Part model, mm, in its own coordinate system. A direction names the side the tool comes from. Round coordinates to 2 decimals unless told otherwise and drop trailing zeros. Loops run counter-clockwise (first coordinate to the right, second up) from the corner with the lowest first, then second, coordinate; pieces in that order, holes last.
(1) Probe probe 1 along X at (y, z) = (-0.3, 0); probe 2 along X at (y, z) = (-2.5, 0); probe 3 along Y at (x, z) = (-8.5, 2). List the from-to ranges inside material, lowest first.
(2) Mould opens along Z. For faces 3 (the face through (0, -1, -5.85)), 4 (the face through (-0.976, -0.507, 0.217)), 5 (the face through (2, -1.95, -4)) say: +Z half, -Z half, draft (parallel to the pull), parting line (faces both ways), or undercut.
(3) Flat gauge pins, fed straight in: pin 1 (3 mm diameter, centred on y = -1, z = 2.5, fed in from +X); pin 2 (1 mm diameter, centred on y = -3.5, z = 2, fed in from +X); pin 3 (3 mm diameter, centred on x = -0.5, z = -1, fed in from -Y). Where does each tip first touch, or does it go through?
(4) Cut at B-B on z = 0. List the corners of the cut face in (x, y).
(5) Tool access for faces 1 (the face through (0, -1, -1.2)), 2 (the face through (11, -1, 0)): list every direction of +Z, -Z, +X, -X, +Y, -Y with a clear straight run to the whole face (end or side of a thin tool).
(6) Cut at C-C on y = -4.95. List the corners of the cut face in (x, z), then the cut area to 3 significant figures.
(7) Cut at D-D on z = -1.5. List the corners of the cut face in (x, y), then the cut area to 3 significant figures.
(8) Cut at A-A on x = 0. List the corners of the cut face in (y, z), then the cut area to 3 significant figures.
from build123d import *

# Parameters (mm, degrees)
BOSS_EXTRUDE1_DEPTH     = 1.95
SKETCH2_R               = 4
BOSS_EXTRUDE2_DEPTH     = 3.55
SKETCH3_R               = 2.86
CUT_EXTRUDE1_DEPTH      = 4.5
SKETCH4_R               = 1
CUT_EXTRUDE2_DEPTH      = 1
CUT_EXTRUDE3_DEPTH      = 25.219723368
CUT_EXTRUDE3_DEPTH_BACK = 25.219723368
SKETCH5_OUTSIDE_W       = 57.198
SKETCH5_OUTSIDE_H       = 23.198
SKETCH5_OUTSIDE_R       = 11


with BuildPart() as part:
    # Sketch1 → Boss-Extrude1 (new body)
    with BuildSketch(Plane(origin=(0, 0, 0), x_dir=(1, 0, 0), z_dir=(0, 1, 0))):
        with BuildLine():
            Line((17, 5.85), (-17, 5.85))
            ThreePointArc((-17, 5.85), (-21.13657467, 4.13657467), (-22.85, 0))
            ThreePointArc((-22.85, 0), (-21.13657467, -4.13657467), (-17, -5.85))
            Line((-17, -5.85), (17, -5.85))
            ThreePointArc((17, -5.85), (21.13657467, -4.13657467), (22.85, 0))
            ThreePointArc((22.85, 0), (21.13657467, 4.13657467), (17, 5.85))
        make_face()
    extrude(amount=-BOSS_EXTRUDE1_DEPTH)

    # Sketch2 → Boss-Extrude2 (add)
    with BuildSketch(Plane.XZ.offset(1.95)):
        with Locations(Location((0, 0, 0), (0, 0, 90))):
            Circle(SKETCH2_R)
    extrude(amount=BOSS_EXTRUDE2_DEPTH)

    # Sketch3 → Cut-Extrude1 (cut)
    with BuildSketch(Plane.XZ.offset(5.5)):
        with Locations(Location((0, 0, 0), (0, 0, 270))):
            Circle(SKETCH3_R)
    extrude(amount=-CUT_EXTRUDE1_DEPTH, mode=Mode.SUBTRACT)

    # Sketch4 → Cut-Extrude2 (cut)
    with BuildSketch(Plane.XZ.offset(1)):
        with Locations(Location((0, 0, 0), (0, 0, 270))):
            Circle(SKETCH4_R)
    extrude(amount=-CUT_EXTRUDE2_DEPTH, mode=Mode.SUBTRACT)

    # Sketch5 outside → Cut-Extrude3 (cut, two sides: drawn at the far end of the back side and taken through both)
    with BuildSketch(Plane(origin=(0, 0, 0), x_dir=(1, 0, 0), z_dir=(0, 1, 0)).offset(-CUT_EXTRUDE3_DEPTH_BACK)):
        Rectangle(SKETCH5_OUTSIDE_W, SKETCH5_OUTSIDE_H)
        Circle(SKETCH5_OUTSIDE_R, mode=Mode.SUBTRACT)
    extrude(amount=CUT_EXTRUDE3_DEPTH + CUT_EXTRUDE3_DEPTH_BACK, mode=Mode.SUBTRACT)


solid = part.part
Final values:
1. probe 1: x = -11 to -1, 1 to 11
1. probe 2: x = -4 to -2.86, 2.86 to 4
1. probe 3: y = -1.95 to 0
2. face 3: -Z half
2. face 4: undercut
2. face 5: draft
3. pin 1: stops at x = 10.95
3. pin 2: stops at x = 3.71
3. pin 3: stops at y = -1
4. outline: (-11, -1.95) - (-4, -1.95) - (-4, -5.5) - (-2.86, -5.5) - (-2.86, -1) - (-1, -1) - (-1, 0) - (-11, 0) - close; (1, -1) - (2.86, -1) - (2.86, -5.5) - (4, -5.5) - (4, -1.95) - (11, -1.95) - (11, 0) - (1, 0) - close
5. face 1: -Y
5. face 2: +X, +Y, -Y
6. outline: circle Ø8 at (0, 0); hole circle Ø5.72 at (0, 0)
6. area: 24.6 mm2
7. outline: (-10.9, -1.95) - (-3.71, -1.95) - (-3.71, -5.5) - (-2.44, -5.5) - (-2.44, -1) - (2.44, -1) - (2.44, -5.5) - (3.71, -5.5) - (3.71, -1.95) - (10.9, -1.95) - (10.9, 0) - (-10.9, 0) - close
7. area: 46.9 mm2
8. outline: (-5.5, -4) - (-1.95, -4) - (-1.95, -5.85) - (0, -5.85) - (0, -1) - (-1, -1) - (-1, -2.86) - (-5.5, -2.86) - close; (-5.5, 2.86) - (-1, 2.86) - (-1, 1) - (0, 1) - (0, 5.85) - (-1.95, 5.85) - (-1.95, 4) - (-5.5, 4) - close
8. area: 23.5 mm2
